from build123d import *

# Parameters (mm, degrees)
F0_W              = 31.75
F0_H              = 31.75
F1_DEPTH          = 38.1
F2_SIZE           = 1.5875
F4_DEPTH          = 31.751
F7_DEPTH          = 12.7
F10_DEPTH         = 12.7
F13_COPIES2_COUNT = 2


# Not quite as in the source:
# - a pattern or mirror of a feature is missing from the dataset's text; its kind, count and spacing are read off the source's solid


with BuildPart() as f1:
    # F0 (on Front) → F1 (new body, symmetric)
    with BuildSketch(Plane.XZ):
        Rectangle(F0_W, F0_H)
    extrude(amount=F1_DEPTH, both=True)

    # F2
    f2_edges = [f1.edges().sort_by_distance(p)[0] for p in [
        (0, -38.1, 15.875),
        (15.875, -38.1, 0),
        (15.875, 0, 15.875),
        (15.875, 0, -15.875),
        (-15.875, 0, 15.875),
        (-15.875, -38.1, 0),
        (0, -38.1, -15.875),
        (15.875, 38.1, 0),
        (-15.875, 38.1, 0),
        (0, 38.1, -15.875),
        (-15.875, 0, -15.875),
        (0, 38.1, 15.875),
    ]]
    chamfer(f2_edges, length=F2_SIZE)

    # F3 (on face) → F4 (cut, through all)
    with BuildSketch(Plane.XY.offset(15.875)):
        with BuildLine():
            Line((11.1125, -12.7), (14.2875, -12.7))
            Line((14.2875, -12.7), (14.2875, 1.197e-07))
            ThreePointArc((14.2875, 1.197e-07), (13.4817207372, -6.5454301226), (11.1125, -12.7))
        make_face()
        Polygon((14.2875, 1.197e-07), (14.2875, -12.7), (15.875, -12.7), (15.875, 12.7), (14.2875, 12.7), align=None)
        with BuildLine():
            ThreePointArc((11.1125, 12.7), (13.4817207082, 6.5454302387), (14.2875, 1.197e-07))
            Line((14.2875, 1.197e-07), (14.2875, 12.7))
            Line((14.2875, 12.7), (11.1125, 12.7))
        make_face()
        Polygon((-15.875, -12.7), (-14.2875, -12.7), (-14.2875, 1.197e-07), (-14.2875, 12.7), (-15.875, 12.7), align=None)
        with BuildLine():
            Line((-14.2875, 1.197e-07), (-14.2875, -12.7))
            Line((-14.2875, -12.7), (-11.1125, -12.7))
            ThreePointArc((-11.1125, -12.7), (-13.4817207372, -6.5454301226), (-14.2875, 1.197e-07))
        make_face()
        with BuildLine():
            Line((-14.2875, 12.7), (-14.2875, 1.197e-07))
            ThreePointArc((-14.2875, 1.197e-07), (-13.4817207082, 6.5454302387), (-11.1125, 12.7))
            Line((-11.1125, 12.7), (-14.2875, 12.7))
        make_face()
        with BuildLine():
            Line((-7.9375, 4.7625), (-7.9375, -4.7625))
            ThreePointArc((-7.9375, -4.7625), (0, -12.7), (7.9375, -4.7625))
            Line((7.9375, -4.7625), (7.9375, 4.7625))
            ThreePointArc((7.9375, 4.7625), (0, 12.7), (-7.9375, 4.7625))
        make_face()
    extrude(amount=-F4_DEPTH, mode=Mode.SUBTRACT)

    # F6 (on face) → F7 (cut, symmetric)
    with BuildSketch(Plane(origin=(0, 0, 0), x_dir=(0, 1, 0), z_dir=(0.7071067812, 0, 0.7071067812))):
        Polygon((-25.4, 18.1531082875), (-22.225, 21.3281082875), (-28.575, 21.3281082875), align=None)
        Polygon((-25.4, -18.1531082875), (-28.575, -21.3281082875), (-22.225, -21.3281082875), align=None)
        Polygon((22.225, -21.3281082875), (28.575, -21.3281082875), (25.4, -18.1531082875), align=None)
        Polygon((28.575, 21.3281082875), (22.225, 21.3281082875), (25.4, 18.1531082875), align=None)
    extrude(amount=F7_DEPTH, both=True, mode=Mode.SUBTRACT)

    # F9 (on face) → F10 (cut, symmetric)
    with BuildSketch(Plane(origin=(0, 0, 0), x_dir=(0, 1, 0), z_dir=(0.7071067812, 0, -0.7071067812))):
        Polygon((-25.4, 18.1531082875), (-22.225, 21.3281082875), (-28.575, 21.3281082875), align=None)
        Polygon((-28.575, -21.3281082875), (-22.225, -21.3281082875), (-25.4, -18.1531082875), align=None)
        Polygon((28.575, 21.3281082875), (22.225, 21.3281082875), (25.4, 18.1531082875), align=None)
        Polygon((25.4, -18.1531082875), (22.225, -21.3281082875), (28.575, -21.3281082875), align=None)
    extrude(amount=F10_DEPTH, both=True, mode=Mode.SUBTRACT)

    # F13: sweep along a path in F11
    with BuildLine(Plane(origin=(-15.875, 0, 0), x_dir=(0, -1, 0), z_dir=(-1, 0, 0))) as f13_path:
        Line((-25.4, 4.4901280605), (-29.8901280605, 0))
        Line((-29.8901280605, 0), (-25.4, -4.4901280605))
        Line((-25.4, -4.4901280605), (-20.9098719395, 0))
        Line((-20.9098719395, 0), (-25.4, 4.4901280605))
    # F12 (on Top) → F13 (sweep, cut)
    with BuildSketch(Plane.XY):
        Polygon((-15.875, 29.4318562844), (-15.08125, 29.8901280605), (-15.875, 30.3483998367), align=None)
    f13 = sweep(path=f13_path.line, transition=Transition.RIGHT, mode=Mode.SUBTRACT)

    # F13_copies: F13 across plane
    add(f13.mirror(Plane(origin=(0, 0, 0), x_dir=(0, 0, 1), z_dir=(1, 0, 0))), mode=Mode.SUBTRACT)

    # F13_copies1: F13 across plane
    add(f13.mirror(Plane(origin=(0, 0, 0), x_dir=(0, 0, -1), z_dir=(0, -1, 0))), mode=Mode.SUBTRACT)

    # F13_copies2: F13 ×2 about axis
    f13_copies2_axis = Axis((0, 0, 0), (0, 0, 1))
    for i in range(1, F13_COPIES2_COUNT):
        add(f13.rotate(f13_copies2_axis, i * 360 / F13_COPIES2_COUNT), mode=Mode.SUBTRACT)


solid = f1.part
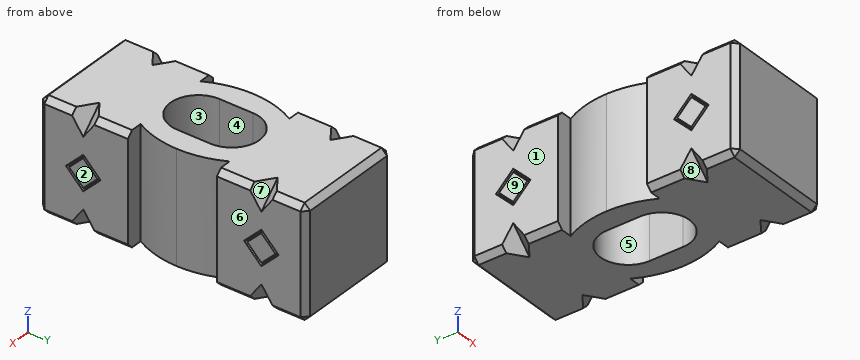
Read the model definition and answer for the solid it produces. Units are mm, in the model's axes. Face numbers are marked on the shaded views. A direction names the side the tool comes from. Coordinates: 2 decimals unless noted, no trailing zeros. Loops run counter-clockwise (first coordinate to the right, second up) from the corner with the lowest first, then second, coordinate; pieces in that order, holes last.
Q1. Consider probe 1 along Y at (x, z) = (0, 0); probe 2 along X at (y, z) = (11.5, 5); probe 3 along Y at (x, z) = (6, -7). Determine where each line is inside the solid, lowest interval first.
Q2. Each of these flat-tipped pins is pushed along its axis until it touches: pin 1 Ø1.5 at (y, z) = (-4, 0.5) entering from -X; pin 2 Ø7.5 at (y, z) = (-2, -2.5) entering from +X; pin 3 Ø3 at (y, z) = (-2.5, -2.5) entering from -X. Where does it stop, or does it pass through?
Q3. The part is cut by section D-D on x = 4.5. Write down the section's boundary in (y, z) (1 decimal).
Q4. The part is cut by section C-C on x = -12. Write down the section's boundary in (y, z) (1 decimal).
Q5. Which of the six approach directions +Z, -Z, +X, -X, +Y, -Y give full straight-line access (tool end or side, diameter ignored) to the marked faces 5, 6, 7, 8 and 9?
Q6. The part is cut by section B-B on z = -7.5. Write down the section's boundary in (x, y) (1 decimal).
Q7. The mould has two halves that part along X. Classify the marked faces 1, 2, 3 and 4: +X half, -X half, draft (parallel to the pull), parting line (faces both ways), or undercut.
Q8. The part is cut by section A-A on x = 0. Write down the section's boundary in (y, z) (1 decimal), and give its area (3 significant figures).
Results below:
1. probe 1: y = -38.1 to -12.7, 12.7 to 38.1
1. probe 2: x = -11.71 to -4.2, 4.2 to 11.71
1. probe 3: y = -38.1 to -9.96, 9.96 to 38.1
2. pin 1: stops at x = -14.09
2. pin 2: stops at x = 14.29
2. pin 3: stops at x = -14.27
3. outline: (-38.1, -14.3) - (-36.5, -15.9) - (-11.3, -15.9) - (-11.3, 15.9) - (-36.5, 15.9) - (-38.1, 14.3) - close; (11.3, -15.9) - (36.5, -15.9) - (38.1, -14.3) - (38.1, 14.3) - (36.5, 15.9) - (11.3, 15.9) - close
4. outline: (-38.1, -14.3) - (-36.5, -15.9) - (-27, -15.9) - (-25.4, -13.7) - (-23.8, -15.9) - (-12.7, -15.9) - (-12.7, 15.9) - (-23.8, 15.9) - (-25.4, 13.7) - (-27, 15.9) - (-36.5, 15.9) - (-38.1, 14.3) - close; (-10.9, -15.9) - (10.9, -15.9) - (10.9, 15.9) - (-10.9, 15.9) - close; (12.7, -15.9) - (23.8, -15.9) - (25.4, -13.7) - (27, -15.9) - (36.5, -15.9) - (38.1, -14.3) - (38.1, 14.3) - (36.5, 15.9) - (27, 15.9) - (25.4, 13.7) - (23.8, 15.9) - (12.7, 15.9) - close
5. face 5: +Z, -Z
5. face 6: +Z, -Z, +X, +Y, -Y
5. face 7: +Z, +X
5. face 8: -Z, -X
5. face 9: +Z, -Z, -X, +Y, -Y
6. outline: (-15.9, -36.5) - (-14.3, -38.1) - (14.3, -38.1) - (15.9, -36.5) - (15.9, -12.7) - (11.1, -12.7) arc R27 ccw to (11.1, 12.7) - (15.9, 12.7) - (15.9, 36.5) - (14.3, 38.1) - (-14.3, 38.1) - (-15.9, 36.5) - (-15.9, 12.7) - (-11.1, 12.7) arc R27 ccw to (-11.1, -12.7) - (-15.9, -12.7) - close; hole (-7.9, -4.8) arc R7.9 ccw to (7.9, -4.8) - (7.9, 4.8) arc R7.9 ccw to (-7.9, 4.8) - close
7. face 1: -X half
7. face 2: +X half
7. face 3: undercut
7. face 4: undercut
8. outline: (-38.1, -14.3) - (-36.5, -15.9) - (-12.7, -15.9) - (-12.7, 15.9) - (-36.5, 15.9) - (-38.1, 14.3) - close; (12.7, -15.9) - (36.5, -15.9) - (38.1, -14.3) - (38.1, 14.3) - (36.5, 15.9) - (12.7, 15.9) - close
8. area: 1,610 mm2
